Could you check a few things on this model? Use its own coordinates, in mm. Face numbers are marked on the shaded views. A direction names the side the tool comes from. Give positions to 0.01 mm unless a question says otherwise; leave off trailing zeros. Order: outer loops, then holes, each group sorted by start corner. A loop starts at its lowest first (then second) coordinate and runs counter-clockwise, first axis right, second up. Notation, with made-up numbers: (6.25, 53.5) -> (65.25, 53.5) arc R19 cw to (65.25, 88.5) -> close; hole circle Ø11 at (-15, -31.5). An arc over 180 degrees is marked (long way). Write each question's results on one line, items separated by ' | '.
```python
from build123d import *

# Parameters (mm, degrees)
SKETCH1_W             = 90
SKETCH1_H             = 40
BASE_FLANGE1_DEPTH    = 0.7
EDGE_FLANGE1_DEPTH    = 50
CUT_EXTRUDE1_REACH    = 72.046
SKETCH7_R             = 1.525
CUT_EXTRUDE2_REACH    = 72.046
SKETCH8_R             = 4.5
CUT_EXTRUDE4_REACH    = 62.893
SKETCH10_R            = 2
BREAK_CORNER6_START   = -21.4
BREAK_CORNER6_DEPTH   = 0.7
BREAK_CORNER6_START_2 = -0.7
BREAK_CORNER6_2_DEPTH = 0.7


# Read off the part's stored shape, not the designer's step: Break-Corner6
# Sheet-metal steps are written as plain solids
with BuildPart() as part:
    # Sketch1 → Base-Flange1 (new body)
    with BuildSketch(Plane(origin=(0, 0, 0), x_dir=(1, 0, 0), z_dir=(0, 1, 0))):
        Rectangle(SKETCH1_W, SKETCH1_H)
    extrude(amount=-BASE_FLANGE1_DEPTH)

    # Edge-Flange1 section (across the edge) → Edge-Flange1 (add)
    with BuildSketch(Plane(origin=(25, 0, -20.7), x_dir=(0, 0, 1), z_dir=(-1, 0, 0))):
        with BuildLine():
            Line((-0.7, 0.7), (-0.7, 35))
            Line((-0.7, 35), (0, 35))
            Line((0, 35), (0, 0.7))
            ThreePointArc((0, 0.7), (0.205025253, 0.205025253), (0.7, 0))
            Line((0.7, 0), (0.7, -0.7))
            ThreePointArc((0.7, -0.7), (-0.289949494, -0.289949494), (-0.7, 0.7))
        make_face()
    extrude(amount=EDGE_FLANGE1_DEPTH)

    # Sketch7 → Cut-Extrude1 (cut, up to next)
    with BuildSketch(Plane.XY.offset(-20.7), mode=Mode.PRIVATE) as cut_extrude1_sk1:
        with Locations((0, 30.02483)):
            Circle(SKETCH7_R)
    cut_extrude1_tool1 = extrude(cut_extrude1_sk1.sketch, amount=-CUT_EXTRUDE1_REACH, mode=Mode.PRIVATE) & part.part
    # Sketch7 → Cut-Extrude1 (cut, up to next)
    with BuildSketch(Plane.XY.offset(-20.7), mode=Mode.PRIVATE) as cut_extrude1_sk2:
        with Locations((10.2108, 7.85063)):
            Circle(SKETCH7_R)
    cut_extrude1_tool2 = extrude(cut_extrude1_sk2.sketch, amount=-CUT_EXTRUDE1_REACH, mode=Mode.PRIVATE) & part.part
    # Sketch7 → Cut-Extrude1 (cut, up to next)
    with BuildSketch(Plane.XY.offset(-20.7), mode=Mode.PRIVATE) as cut_extrude1_sk3:
        with Locations((-10.2108, 7.85063)):
            Circle(SKETCH7_R)
    cut_extrude1_tool3 = extrude(cut_extrude1_sk3.sketch, amount=-CUT_EXTRUDE1_REACH, mode=Mode.PRIVATE) & part.part
    add(cut_extrude1_tool1.solids().sort_by_distance((0, 30.02483, -20.7))[0], mode=Mode.SUBTRACT)
    add(cut_extrude1_tool2.solids().sort_by_distance((10.2108, 7.85063, -20.7))[0], mode=Mode.SUBTRACT)
    add(cut_extrude1_tool3.solids().sort_by_distance((-10.2108, 7.85063, -20.7))[0], mode=Mode.SUBTRACT)

    # Sketch8 → Cut-Extrude2 (cut, up to next)
    with BuildSketch(Plane.XY.offset(-20.7), mode=Mode.PRIVATE) as cut_extrude2_sk1:
        with Locations((0, 7.85063)):
            Circle(SKETCH8_R)
    cut_extrude2_tool1 = extrude(cut_extrude2_sk1.sketch, amount=-CUT_EXTRUDE2_REACH, mode=Mode.PRIVATE) & part.part
    add(cut_extrude2_tool1.solids().sort_by_distance((0, 7.85063, -20.7))[0], mode=Mode.SUBTRACT)

    # Sketch10 → Cut-Extrude4 (cut, up to next)
    with BuildSketch(Plane(origin=(0, 0, 0), x_dir=(1, 0, 0), z_dir=(0, 1, 0)), mode=Mode.PRIVATE) as cut_extrude4_sk1:
        with Locations(Location((-40.378, -7.5, 0), (0, 0, 270))):
            Circle(SKETCH10_R)
    cut_extrude4_tool1 = extrude(cut_extrude4_sk1.sketch, amount=-CUT_EXTRUDE4_REACH, mode=Mode.PRIVATE) & part.part
    # Sketch10 → Cut-Extrude4 (cut, up to next)
    with BuildSketch(Plane(origin=(0, 0, 0), x_dir=(1, 0, 0), z_dir=(0, 1, 0)), mode=Mode.PRIVATE) as cut_extrude4_sk2:
        with Locations(Location((40.378, -7.5, 0), (0, 0, 270))):
            Circle(SKETCH10_R)
    cut_extrude4_tool2 = extrude(cut_extrude4_sk2.sketch, amount=-CUT_EXTRUDE4_REACH, mode=Mode.PRIVATE) & part.part
    add(cut_extrude4_tool1.solids().sort_by_distance((-40.378, 0, 7.5))[0], mode=Mode.SUBTRACT)
    add(cut_extrude4_tool2.solids().sort_by_distance((40.378, 0, 7.5))[0], mode=Mode.SUBTRACT)

    # Break-Corner6 outline → Break-Corner6 (cut)
    with BuildSketch(Plane.XY.offset(BREAK_CORNER6_START)):
        with BuildLine():
            ThreePointArc((-25, 30), (-23.535533906, 33.535533906), (-20, 35))
            Line((-20, 35), (-25, 35))
            Line((-25, 35), (-25, 30))
        make_face()
        with BuildLine():
            ThreePointArc((20, 35), (23.535533906, 33.535533906), (25, 30))
            Line((25, 30), (25, 35))
            Line((25, 35), (20, 35))
        make_face()
    extrude(amount=BREAK_CORNER6_DEPTH, mode=Mode.SUBTRACT)

    # Break-Corner6 2 outline → Break-Corner6 2 (cut)
    with BuildSketch(Plane(origin=(0, 0, 0), x_dir=(1, 0, 0), z_dir=(0, 1, 0)).offset(BREAK_CORNER6_START_2)):
        with BuildLine():
            ThreePointArc((40, 20), (43.535533906, 18.535533906), (45, 15))
            Line((45, 15), (45, 20))
            Line((45, 20), (40, 20))
        make_face()
        with BuildLine():
            Line((-45, 20), (-45, 15))
            ThreePointArc((-45, 15), (-43.535533906, 18.535533906), (-40, 20))
            Line((-40, 20), (-45, 20))
        make_face()
        with BuildLine():
            Line((-45, -20), (-40, -20))
            ThreePointArc((-40, -20), (-43.535533906, -18.535533906), (-45, -15))
            Line((-45, -15), (-45, -20))
        make_face()
        with BuildLine():
            ThreePointArc((45, -15), (43.535533906, -18.535533906), (40, -20))
            Line((40, -20), (45, -20))
            Line((45, -20), (45, -15))
        make_face()
    extrude(amount=BREAK_CORNER6_2_DEPTH, mode=Mode.SUBTRACT)


solid = part.part
```
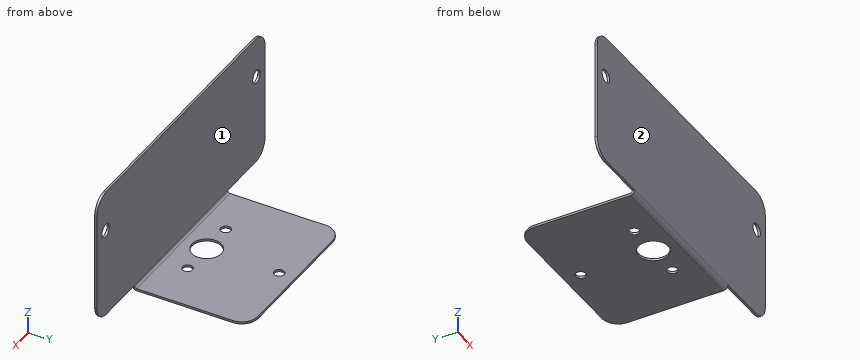
Q1. I need wall thicknesses on line 1 along X through (y, z) = (-0.15, 7.5); line 2 along Y through (x, z) = (0, -21.2); line 3 along Y through (x, z) = (0, -21.1). Which ranges of each line are inside material? Lowest first, please.
Here are the results:
line 1: x = -45 to -42.38, -38.38 to 38.38, 42.38 to 45 | line 2: y = -0.02 to 3.35, 12.35 to 28.5, 31.55 to 35 | line 3: y = -0.17 to 3.35, 12.35 to 28.5, 31.55 to 35
Q2. Suppose I cut it at B-B on x = 0. Please give me the cut outline in (y, z), and give its area (3 significant figures).
Here are the results:
outline: (-0.7, -20) arc R1.4 ccw to (0.7, -21.4) -> (3.35, -21.4) -> (3.35, -20.7) -> (0.7, -20.7) arc R0.7 cw to (0, -20) -> (0, 20) -> (-0.7, 20) -> close; (12.35, -21.4) -> (28.5, -21.4) -> (28.5, -20.7) -> (12.35, -20.7) -> close; (31.55, -21.4) -> (35, -21.4) -> (35, -20.7) -> (31.55, -20.7) -> close | area: 44.7 mm²
Q3. Suppose I cut it at D-D on x = -15. Please give me the cut outline in (y, z).
Here are the results:
outline: (-0.7, -20) arc R1.4 ccw to (0.7, -21.4) -> (35, -21.4) -> (35, -20.7) -> (0.7, -20.7) arc R0.7 cw to (0, -20) -> (0, 20) -> (-0.7, 20) -> close
Q4. Suppose I cut it at A-A on z = 7.5. Please give me the cut outline in (x, y).
Here are the results:
outline: (-45, -0.7) -> (-42.38, -0.7) -> (-42.38, 0) -> (-45, 0) -> close; (-38.38, -0.7) -> (38.38, -0.7) -> (38.38, 0) -> (-38.38, 0) -> close; (42.38, -0.7) -> (45, -0.7) -> (45, 0) -> (42.38, 0) -> close
Q5. I'm going to push flat-ended pins straight in: pin 1 Ø2.5 at (x, z) = (40.378, 7.5) entering from -Y; pin 2 Ø12 at (x, z) = (-3, -10) entering from +Y; pin 3 Ø17 at (x, y) = (-1, 11.5) entering from +Z; pin 4 Ø0.7 at (y, z) = (10, -21) entering from +X. Where does each tip first touch, or does it pass through?
Here are the results:
pin 1: passes through | pin 2: stops at y = 0 | pin 3: stops at z = -20.7 | pin 4: stops at x = 25
Q6. For the marked faces 1 and 2, which set-ups out of +Z, -Z, +X, -X, +Y, -Y let a thin tool reach every point of the face, with its end or its side?
Here are the results:
face 1: +Z, +X, -X, +Y | face 2: +Z, -Z, +X, -X, -Y
Q7. Suppose I cut it at C-C on y = 11. Please give me the cut outline in (x, z).
Here are the results:
outline: (-25, -21.4) -> (-3.21, -21.4) -> (-3.21, -20.7) -> (-25, -20.7) -> close; (3.21, -21.4) -> (25, -21.4) -> (25, -20.7) -> (3.21, -20.7) -> close
